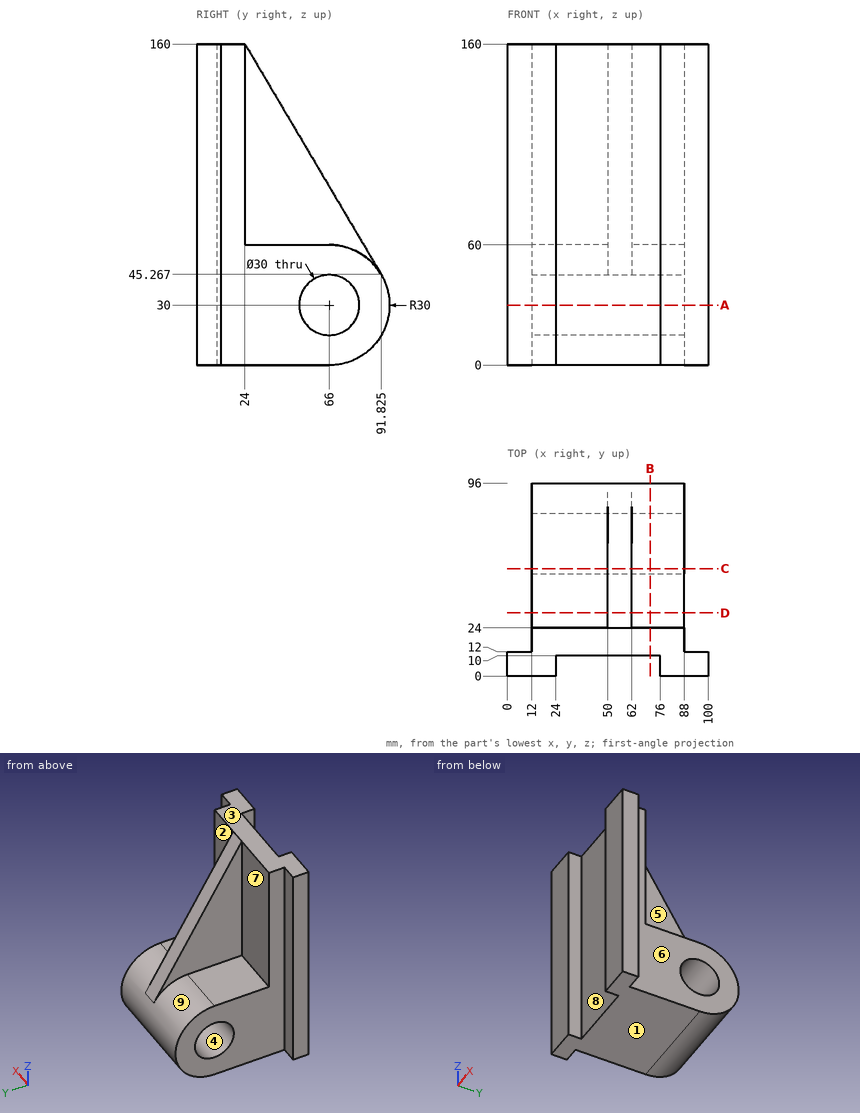
Can you work these out from the drawing? Everything is in mm from the part's minimum corner. A direction names the side the tool comes from. Coordinates: 2 decimals unless noted, no trailing zeros. Write each loop counter-clockwise with the first axis right and the second up, starting at its lowest first coordinate (ties: lowest second). Pieces come first, ordered by that corner, then holes. Notation, with made-up numbers: (82, -29) - (131, -29) arc R21 ccw to (131, -21) - close; hole circle Ø10 at (-11.75, 70.25). An arc over 180 degrees is marked (long way). Use a Markdown table: item, result.
Q1. Which directions (+Z, -Z, +X, -X, +Y, -Y) give clear straight access to the entire face, cutting with the end or side of a thin tool? Please do the marked faces 5, 6, 7, 8 and 9.
Geometry check:
| item | result |
|---|---|
| face 5 | +Z, +X, +Y |
| face 6 | +Z, -Z, +X, +Y |
| face 7 | +Z, -X, +Y |
| face 8 | +Z, -Z, -Y |
| face 9 | +Y |
Q2. Imagine slicing it at D-D (y = 31.5). List the corners of the cut face in (x, z) for me.
Geometry check:
| item | result |
|---|---|
| outline | (12, 0) - (88, 0) - (88, 60) - (62, 60) - (62, 147.31) - (50, 147.31) - (50, 60) - (12, 60) - close |
Q3. Imagine slicing it at A-A (z = 30). List the corners of the cut face in (x, y) for me, and give its area (3 significant figures).
Geometry check:
| item | result |
|---|---|
| outline | (0, 0) - (24, 0) - (24, 10) - (76, 10) - (76, 0) - (100, 0) - (100, 12) - (88, 12) - (88, 51) - (12, 51) - (12, 12) - (0, 12) - close; (12, 81) - (88, 81) - (88, 96) - (12, 96) - close |
| area | 4,780 mm2 |
Q4. Please list where these lines run through material, in increasing order: L1, parallel to Y at x = 40, z = 30; L2, parallel to X at y = 51, z = 72; L3, parallel to Y at x = 39.5, z = 128.5.
Geometry check:
| item | result |
|---|---|
| L1 | y = 10 to 51, 81 to 96 |
| L2 | x = 50 to 62 |
| L3 | y = 10 to 24 |
Q5. Imagine slicing it at B-B (x = 71). List the corners of the cut face in (y, z) for me.
Geometry check:
| item | result |
|---|---|
| outline | (10, 0) - (66, 0) arc R30 ccw to (66, 60) - (24, 60) - (24, 160) - (10, 160) - close; hole circle Ø30 at (66, 30) |
Q6. Thinking about a two-plate mould opening in Z: for the marked faces 1, 2, 3 and 4, which applies, +Z half, -Z half, draft (parallel to the pull), parting line (faces both ways), or undercut?
Geometry check:
| item | result |
|---|---|
| face 1 | -Z half |
| face 2 | draft |
| face 3 | +Z half |
| face 4 | undercut |
Q7. Imagine slicing it at C-C (y = 53.5). List the corners of the cut face in (x, z) for me.
Geometry check:
| item | result |
|---|---|
| outline | (12, 0) - (88, 0) - (88, 21.71) - (12, 21.71) - close; (12, 38.29) - (88, 38.29) - (88, 60) - (62, 60) - (62, 110.1) - (50, 110.1) - (50, 60) - (12, 60) - close |
Q8. I'm going to push flat-ended pins straight in: pin 1 Ø21 at (x, y) = (75, 43) entering from +Z; pin 2 Ø3 at (y, z) = (29.5, 74) entering from -X; pin 3 Ø1 at (y, z) = (15, 49.5) entering from +X. Where does each tip first touch, or does it pass through?
Geometry check:
| item | result |
|---|---|
| pin 1 | stops at z = 60 |
| pin 2 | stops at x = 50 |
| pin 3 | stops at x = 88 |
